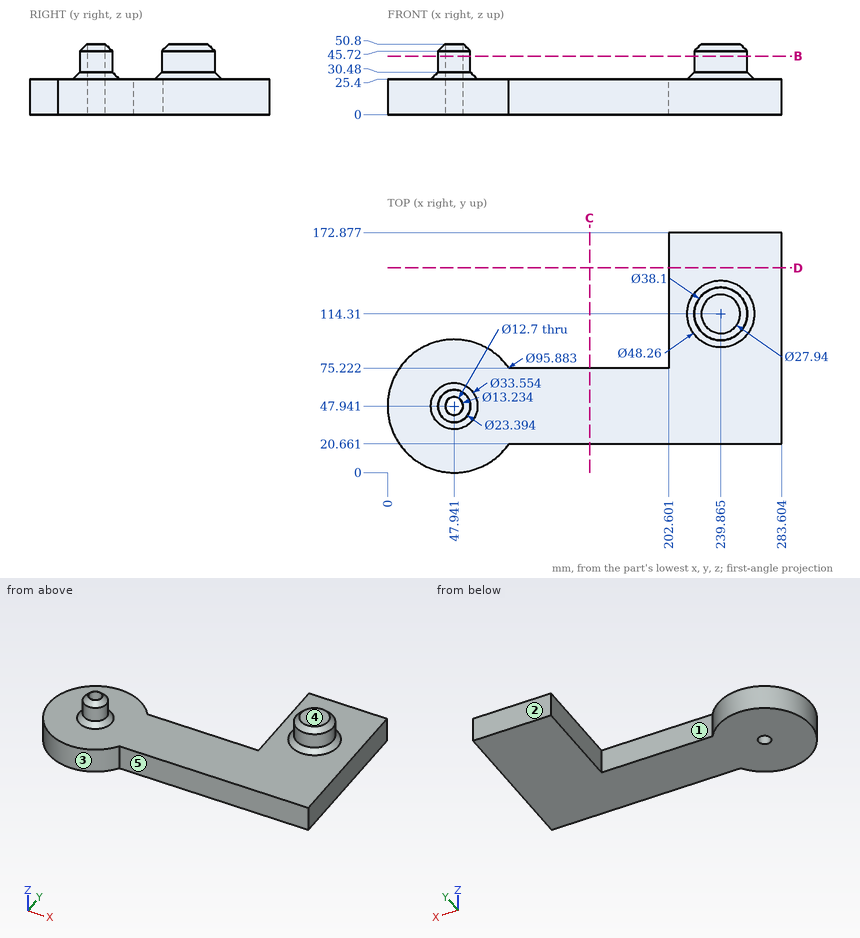
The figure shows three views and two pictorial views of one solid part (mm, origin at its lowest corner). Answer the questions. A direction names the side the tool comes from. Round coordinates to 2 decimals unless told otherwise and drop trailing zeros. Order: outer loops, then holes, each group sorted by start corner. A loop starts at its lowest first (then second) coordinate and runs counter-clockwise, first axis right, second up.
Q1. The mould has two halves that part along X. Classify the marked faces 1, 2 and 3: pulls with the +X half, pulls with the -X half, needs draft (parallel to the pull), parting line crosses it, or undercut.
Solution:
face 1: undercut
face 2: needs draft
face 3: undercut
Q2. A cutting plane is placed at D-D, the plane y = 147.5. Determine the outline of the cut face in (x, z), then the cut area to 3 significant figures.
Solution:
outline: (202.6, 0) - (283.6, 0) - (283.6, 25.4) - (202.6, 25.4) - close
area: 2,060 mm2
Q3. A cutting plane is placed at C-C, the plane x = 145.5. Determine the outline of the cut face in (y, z), then the cut area to 3 significant figures.
Solution:
outline: (20.66, 0) - (75.22, 0) - (75.22, 25.4) - (20.66, 25.4) - close
area: 1,390 mm2
Q4. Given pin 1 Ø3 at (x, z) = (60, 19.5) entering from -Y; pin 2 Ø20.5 at (y, z) = (130, 14.5) entering from -X; pin 3 Ø7.5 at (x, z) = (162, 18.5) entering from -Y, each flat-ended and moving along its own axis, determine where each tip first touches the part or whether it passes through.
Solution:
pin 1: stops at y = 1.18
pin 2: stops at x = 202.6
pin 3: stops at y = 20.66
Q5. A cutting plane is placed at B-B, the plane z = 42. Count the separate pieces of the cut face and the enclosed holes in it, then the cut area to 3 significant figures.
Solution:
separate pieces: 2
enclosed holes: 1
area: 1,440 mm2
Q6. A tool of negligible diameter and unlimited length cuts with its end or side. For the marked faces 4 and 5, from which of +Z, -Z, +X, -X, +Y, -Y can it reach the whole face along a straight path? Write none if from no direction.
Solution:
face 4: +Z, +X, -X, +Y, -Y
face 5: +Z, -Z, +X, -Y
Q7. Find the intervals of material crossed by line 1 along X through (y, z) = (47.5, 15) (1 decimal); line 2 along Z through (x, y) = (249.5, 91.5); line 3 along Y through (x, z) = (51, 15) (1 decimal), in increasing order.
Solution:
line 1: x = 0 to 41.6, 54.3 to 283.6
line 2: z = 0 to 25.4
line 3: y = 0.1 to 42.4, 53.5 to 95.8
